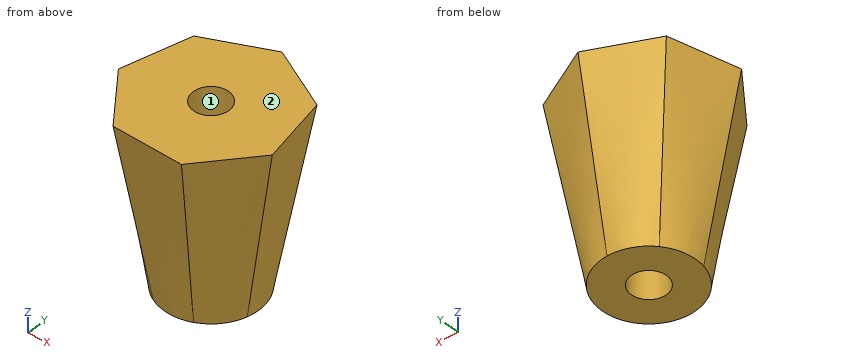
from build123d import *

# Parameters (mm, degrees)
F4_R     = 15
F5_DEPTH = 172


# Not quite as in the source:
# - the arcs of a loft's sections are written as splines that run evenly, so that the points pair up as in the source's solid


with BuildPart() as f3:
    # F1 (on Top) → F3 section 0
    with BuildSketch(Plane.XY):
        with BuildLine():
            add(Edge.make_bspline(
                [(31.2732592987, 24.9395920743), (28.7859564656, 28.0585711749), (25.8289364984, 30.8022847428), (19.2366681467, 35.2968172025), (15.6022965087, 37.0470383387), (7.9781174442, 39.3987861242), (3.9893240046, 40), (0, 40)],
                knots=[0, 0, 0, 0, 0.3333333333, 0.3333333333, 0.6666666667, 0.6666666667, 1, 1, 1, 1], degree=3))
            add(Edge.make_bspline(
                [(0, 40), (-3.9893240046, 40), (-7.9781174442, 39.3987861242), (-15.6022965087, 37.0470383387), (-19.2366681467, 35.2968172025), (-25.8289364984, 30.8022847428), (-28.7859564656, 28.0585711749), (-31.2732592987, 24.9395920743)],
                knots=[0, 0, 0, 0, 0.3333333333, 0.3333333333, 0.6666666667, 0.6666666667, 1, 1, 1, 1], degree=3))
            add(Edge.make_bspline(
                [(-31.2732592987, 24.9395920743), (-33.7605621319, 21.8206129738), (-35.7774862274, 18.3271979653), (-38.6924136641, 10.900083984), (-39.590029331, 6.967372789), (-40.1862744435, -0.9889653021), (-39.8848245906, -5.0115340355), (-38.9971164873, -8.9008373583)],
                knots=[0, 0, 0, 0, 0.3333333333, 0.3333333333, 0.6666666667, 0.6666666667, 1, 1, 1, 1], degree=3))
            add(Edge.make_bspline(
                [(-38.9971164873, -8.9008373583), (-38.1094083839, -12.790140681), (-36.6356781537, -16.5451440681), (-32.6463541491, -23.4548559319), (-30.1312909397, -26.6086454432), (-24.282528082, -32.0355043032), (-20.9496062968, -34.3078519004), (-17.3553495647, -36.0387547161)],
                knots=[0, 0, 0, 0, 0.3333333333, 0.3333333333, 0.6666666667, 0.6666666667, 1, 1, 1, 1], degree=3))
            add(Edge.make_bspline(
                [(-17.3553495647, -36.0387547161), (-13.7610928326, -37.7696575317), (-9.9064571986, -38.9586551589), (-2.0169240955, -40.1478109392), (2.0169240955, -40.1478109392), (9.9064571986, -38.9586551589), (13.7610928326, -37.7696575317), (17.3553495647, -36.0387547161)],
                knots=[0, 0, 0, 0, 0.3333333333, 0.3333333333, 0.6666666667, 0.6666666667, 1, 1, 1, 1], degree=3))
            add(Edge.make_bspline(
                [(17.3553495647, -36.0387547161), (20.9496062968, -34.3078519004), (24.282528082, -32.0355043032), (30.1312909397, -26.6086454432), (32.6463541491, -23.4548559319), (36.6356781537, -16.5451440681), (38.1094083839, -12.790140681), (38.9971164873, -8.9008373583)],
                knots=[0, 0, 0, 0, 0.3333333333, 0.3333333333, 0.6666666667, 0.6666666667, 1, 1, 1, 1], degree=3))
            add(Edge.make_bspline(
                [(38.9971164873, -8.9008373583), (39.8848245906, -5.0115340355), (40.1862744435, -0.9889653021), (39.590029331, 6.967372789), (38.6924136641, 10.900083984), (35.7774862274, 18.3271979653), (33.7605621319, 21.8206129738), (31.2732592987, 24.9395920743)],
                knots=[0, 0, 0, 0, 0.3333333333, 0.3333333333, 0.6666666667, 0.6666666667, 1, 1, 1, 1], degree=3))
        make_face()
    # F2 (on offset) → F3 section 1
    with BuildSketch(Plane.XY.offset(150)):
        Polygon((52.9471102464, 42.2239114397), (0, 67.7218958735), (-52.9471102464, 42.2239114397), (-66.023966553, -15.0695395191), (-29.3834294017, -61.0153198574), (29.3834294017, -61.0153198574), (66.023966553, -15.0695395191), align=None)
    loft(ruled=True)

    # F4 (on face) → F5 (cut)
    with BuildSketch(Plane(origin=(0, 0, 0), x_dir=(1, 0, 0), z_dir=(0, 0, -1))):
        Circle(F4_R)
    extrude(amount=-F5_DEPTH, mode=Mode.SUBTRACT)


solid = f3.part
Design review of the part built by this model. Coordinates are the model's own, in mm. Face numbers are marked on the shaded views. Coordinates: 2 decimals unless noted, no trailing zeros. One line per item, written item: value.
1) To check wall thickness, follow probe 1 along X at (y, z) = (0, 102); probe 2 along Y at (x, z) = (0, 45); probe 3 along X at (y, z) = (0, 114). State the ranges of each line that lie inside material, in increasing order.
Answer sheet:
probe 1: x = -55.38 to -15, 15 to 55.38
probe 2: y = -46.3 to -15, 15 to 48.32
probe 3: x = -57.19 to -15, 15 to 57.19
2) Mouldability with a two-part tool opening along Y and no side actions: class the marked faces 1 and 2 as +Y half, -Y half, draft (parallel to the pull), parting line (faces both ways), or undercut.
Answer sheet:
face 1: undercut
face 2: draft
3) Insertion check: pin 1 (8 mm diameter, centred on y = -8, z = 110.5, fed in from -X); pin 2 (2 mm diameter, centred on y = 4.5, z = 41.5, fed in from -X); pin 3 (3 mm diameter, centred on x = -40, y = 3, fed in from -Z); pin 4 (5 mm diameter, centred on x = 12.5, z = 134.5, fed in from +Y). Each pin has a flat end and moves straight along its axis. Give the tip position at first contact, or say it passes through.
Answer sheet:
pin 1: stops at x = -58.99
pin 2: stops at x = -45.95
pin 3: stops at z = 0
pin 4: stops at y = 60.4
